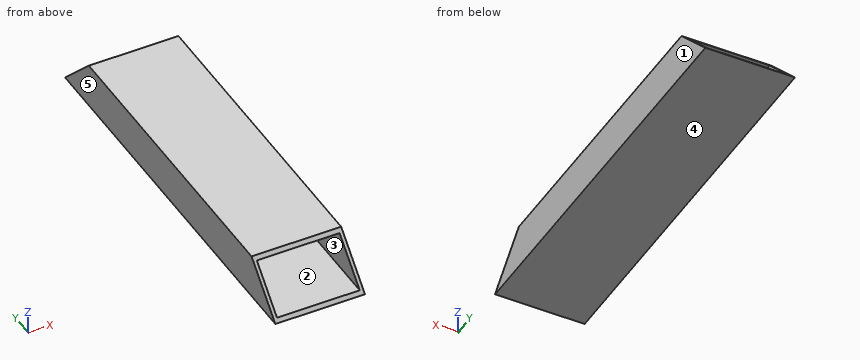
Autodesk Inventor part; units mm, degrees
ref_plane "YZ Plane" through (0, 0, 0) normal (1, 0, 0) x (0, 1, 0)
ref_plane "XZ Plane" through (0, 0, 0) normal (0, 1, 0) x (-1, 0, 0)
ref_plane "XY Plane" through (0, 0, 0) normal (0, 0, 1) x (1, 0, 0)
sketch "スケッチ1" plane through (0, 0, 0) normal (0, 1, 0) x (-1, 0, 0)
  line L0 (-30, 15) -> (30, 15)
  line L1 (30, 15) -> (30, -15)
  line L2 (30, -15) -> (-30, -15)
  line L3 (-30, -15) -> (-30, 15)
  line L4 (-30, 15) -> (30, -15) construction
  line L5 (30, 15) -> (-30, -15) construction
  line L6 (27.7, -12.7) -> (27.7, 12.7)
  line L7 (27.7, 12.7) -> (-27.7, 12.7)
  line L8 (-27.7, 12.7) -> (-27.7, -12.7)
  line L9 (-27.7, -12.7) -> (27.7, -12.7)
  point P0 (0, 0)
  dimension "d0" = 60
  dimension "d1" = 30
  dimension "d2" = 2.3
extrude "押し出し1" add sketch "スケッチ1" along normal mid plane 265
chamfer "面取り1" distance 30 angle 45 2 edges at (0, 132.5, 15) (0, -132.5, 15)
properties part number "車輪受け"
The model under review builds one solid part; all positions refer to its coordinate system, in mm. Face numbers are marked on the shaded views. A direction names the side the tool comes from. Give positions to 0.01 mm unless a question says otherwise; leave off trailing zeros. Write each loop counter-clockwise with the first axis right and the second up, starting at its lowest first coordinate (ties: lowest second). Pieces come first, ordered by that corner, then holes. Notation, with made-up numbers: (83.25, -1) -> (133.25, -1) arc R28 cw to (133.25, 17) -> close; hole circle Ø11 at (28.5, 23.25). An arc over 180 degrees is marked (long way). Answer in a Markdown table with one row per item.
1) Add section A-A on z = 6. State the section outline as (x, y) points, plus the area to 3 significant figures.
Worked answers:
| item | result |
|---|---|
| outline | (-30, -111.5) -> (-27.7, -111.5) -> (-27.7, 111.5) -> (-30, 111.5) -> close; (27.7, -111.5) -> (30, -111.5) -> (30, 111.5) -> (27.7, 111.5) -> close |
| area | 1,030 mm² |
2) Mouldability with a two-part tool opening along X and no side actions: class the marked faces 3, 4 and 5 as +X half, -X half, draft (parallel to the pull), parting line (faces both ways), or undercut.
Worked answers:
| item | result |
|---|---|
| face 3 | undercut |
| face 4 | draft |
| face 5 | -X half |
3) Add section D-D on y = -24.5. State the section outline as (x, z) points, plus the area to 3 significant figures.
Worked answers:
| item | result |
|---|---|
| outline | (-30, -15) -> (30, -15) -> (30, 15) -> (-30, 15) -> close; hole (-27.7, -12.7) -> (27.7, -12.7) -> (27.7, 12.7) -> (-27.7, 12.7) -> close |
| area | 393 mm² |
4) Tool access review of the marked faces 1 and 2: name each direction out of +Z, -Z, +X, -X, +Y, -Y from which nothing blocks a thin tool from reaching the whole face with its end or side.
Worked answers:
| item | result |
|---|---|
| face 1 | +Z, -Z, +X, +Y, -Y |
| face 2 | +Y, -Y |
5) Add section B-B on x = 11. State the section outline as (y, z) points, plus the area to 3 significant figures.
Worked answers:
| item | result |
|---|---|
| outline | (-132.5, -15) -> (132.5, -15) -> (130.2, -12.7) -> (-130.2, -12.7) -> close; (-104.8, 12.7) -> (104.8, 12.7) -> (102.5, 15) -> (-102.5, 15) -> close |
| area | 1,080 mm² |
6) Add section C-C on y = -113. State the section outline as (x, z) points.
Worked answers:
| item | result |
|---|---|
| outline | (-30, -15) -> (30, -15) -> (30, 4.5) -> (27.7, 4.5) -> (27.7, -12.7) -> (-27.7, -12.7) -> (-27.7, 4.5) -> (-30, 4.5) -> close |
7) For L1, parallel to Z at x = -8, y = -9; L2, parallel to X at y = 71.5, z = -5.5; L3, parallel to Z at x = 23.5, y = -107.5, list the stretches that pass through material, from the lowest coordinate up. Write a range as [from, to].
Worked answers:
| item | result |
|---|---|
| L1 | [-15, -12.7], [12.7, 15] |
| L2 | [-30, -27.7], [27.7, 30] |
| L3 | [-15, -12.7] |
